Model file for the job. Use its own axes, mm. A direction names the side the tool comes from. Give positions to 0.01 mm unless a question says otherwise; leave off trailing zeros. Loops run counter-clockwise (first coordinate to the right, second up) from the corner with the lowest first, then second, coordinate; pieces in that order, holes last. Notation, with made-up numbers: (57, 1.25) - (78, 1.25) arc R19 cw to (78, 20.25) - close; hole circle Ø6 at (31, 48). An arc over 180 degrees is marked (long way). Use a Markdown table: item, result.
from build123d import *

# Parameters (mm, degrees)
F0_R            = 29.5
F2_DEPTH        = 2.1
F4_DEPTH        = 2.1
F4_COPIES_COUNT = 3
F4_COPIES_ANGLE = 180
F6_DEPTH        = 2.1
F8_DEPTH        = 5.45


# Not quite as in the source:
# - a pattern or mirror of a feature is missing from the dataset's text; its kind, count and spacing are read off the source's solid


with BuildPart() as f2:
    # F0 (on Top) → F2 (new body)
    with BuildSketch(Plane.XY):
        Circle(F0_R)
    extrude(amount=F2_DEPTH)

    # F3 (on face) → F4 (cut, through all)
    with BuildSketch(Plane.XY.offset(2.1)):
        with BuildLine():
            ThreePointArc((-1.7, 27.8), (0, 26.1), (1.7, 27.8))
            Line((1.7, 27.8), (1.7, 29.4509762147))
            ThreePointArc((1.7, 29.4509762147), (0, 29.5), (-1.7, 29.4509762147))
            Line((-1.7, 29.4509762147), (-1.7, 27.8))
        make_face()
    f4 = extrude(amount=-F4_DEPTH, mode=Mode.SUBTRACT)

    # F4_copies: F4 ×3 about axis
    f4_copies_axis = Axis((0, 0, 0), (0, 0, 1))
    for i in range(1, F4_COPIES_COUNT):
        add(f4.rotate(f4_copies_axis, i * F4_COPIES_ANGLE / (F4_COPIES_COUNT - 1)), mode=Mode.SUBTRACT)

    # F5 (on face) → F6 (cut, through all)
    with BuildSketch(Plane.XY.offset(2.1)):
        with BuildLine():
            ThreePointArc((-3, 0.75), (-3.75, 0), (-3, -0.75))
            Line((-3, -0.75), (29.4904645606, -0.75))
            ThreePointArc((29.4904645606, -0.75), (29.5, 0), (29.4904645606, 0.75))
            Line((29.4904645606, 0.75), (-3, 0.75))
        make_face()
    extrude(amount=-F6_DEPTH, mode=Mode.SUBTRACT)

    # F7 (on face) → F8 (join)
    with BuildSketch(Plane(origin=(0, 0, 0), x_dir=(1, 0, 0), z_dir=(0, 0, -1))):
        with BuildLine():
            Line((22.9877684867, 0.75), (24.78865668, 0.75))
            ThreePointArc((24.78865668, 0.75), (-24.8, 0), (24.78865668, -0.75))
            Line((24.78865668, -0.75), (22.9877684867, -0.75))
            ThreePointArc((22.9877684867, -0.75), (-23, 0), (22.9877684867, 0.75))
        make_face()
    extrude(amount=F8_DEPTH)


solid = f2.part
(1) Slice it at D-D, the plane x = -22. Write the cut outline in (y, z), plus the area to 3 significant figures.
Computed:
| item | result |
|---|---|
| outline | (-19.65, 0) - (-11.45, 0) - (-11.45, -5.45) - (-6.71, -5.45) - (-6.71, 0) - (6.71, 0) - (6.71, -5.45) - (11.45, -5.45) - (11.45, 0) - (19.65, 0) - (19.65, 2.1) - (-19.65, 2.1) - close |
| area | 134 mm² |
(2) Slice it at B-B, the plane y = 0. Write the cut outline in (x, z), plus the area to 3 significant figures.
Computed:
| item | result |
|---|---|
| outline | (-26.1, 0) - (-24.8, 0) - (-24.8, -5.45) - (-23, -5.45) - (-23, 0) - (-3.75, 0) - (-3.75, 2.1) - (-26.1, 2.1) - close |
| area | 56.7 mm² |
(3) 3-axis set-ups, long thin cutter, end or side, ignore diameter. For faces 5 (the flat face through (17, 0.75, 1)), 6 (the flat face through (1.7, 29, 1)), 7 (the cylindrical face through (-22.98, 1, -2.69)): which of +Z, -Z, +X, -X, +Y, -Y reach the whole face in a straight line?
Computed:
| item | result |
|---|---|
| face 5 | +Z, -Z, +X |
| face 6 | +Z, -Z, +Y |
| face 7 | -Z |
(4) Pin check, flat tips, straight feed: P1, Ø4, axis at x = 15.5, z = -1, coming from the -Y side; P2, Ø4, axis at y = 15, z = -4.5, coming from the -X side; P3, Ø2, axis at y = -15.5, z = -3.5, coming from the -X side. Stop position of each tip, or through.
Computed:
| item | result |
|---|---|
| P1 | y = -26.09 |
| P2 | x = -21.12 |
| P3 | x = -20.12 |
(5) Drill centre lines: probe 1 along Y at (x, z) = (0, -3.6); probe 2 along Z at (x, y) = (-2, 12); probe 3 along Y at (x, z) = (5, -2.75). Where is each one in solid material? Low to high. Write a range as [from, to].
Computed:
| item | result |
|---|---|
| probe 1 | [-24.8, -23], [23, 24.8] |
| probe 2 | [0, 2.1] |
| probe 3 | [-24.29, -22.45], [22.45, 24.29] |
(6) Slice it at C-C, the plane z = 1.25. Write the cut outline in (x, y), plus the area to 3 significant figures.
Computed:
| item | result |
|---|---|
| outline | (-29.45, -1.7) arc R29.5 ccw to (-1.7, -29.45) - (-1.7, -27.8) arc R1.7 cw to (1.7, -27.8) - (1.7, -29.45) arc R29.5 ccw to (29.49, -0.75) - (-3, -0.75) arc R0.75 cw to (-3, 0.75) - (29.49, 0.75) arc R29.5 ccw to (1.7, 29.45) - (1.7, 27.8) arc R1.7 cw to (-1.7, 27.8) - (-1.7, 29.45) arc R29.5 ccw to (-29.45, 1.7) - (-27.8, 1.7) arc R1.7 cw to (-27.8, -1.7) - close |
| area | 2,650 mm² |
(7) Mould opens along Y. For faces 1 (the flat face through (-7, 24, 0)), 2 (the cylindrical face through (20.98, -20.74, 1.04)), 3 (the cylindrical face through (0, 26.1, 1.1)), 4 (the cylindrical face through (-3.75, 0.02, 1.06)) say: pulls with the +Y half, pulls with the -Y half, needs draft (parallel to the pull), parting line crosses it, or undercut.
Computed:
| item | result |
|---|---|
| face 1 | needs draft |
| face 2 | pulls with the -Y half |
| face 3 | pulls with the +Y half |
| face 4 | undercut |
(8) Slice it at A-A, the plane x = 0. Write the cut outline in (y, z), plus the area to 3 significant figures.
Computed:
| item | result |
|---|---|
| outline | (-26.1, 0) - (-24.8, 0) - (-24.8, -5.45) - (-23, -5.45) - (-23, 0) - (-0.75, 0) - (-0.75, 2.1) - (-26.1, 2.1) - close; (0.75, 0) - (23, 0) - (23, -5.45) - (24.8, -5.45) - (24.8, 0) - (26.1, 0) - (26.1, 2.1) - (0.75, 2.1) - close |
| area | 126 mm² |
